Could you check a few things on this model? Use its own coordinates, in mm. A direction names the side the tool comes from. Round coordinates to 2 decimals unless told otherwise and drop trailing zeros. Write each loop counter-clockwise with the first axis right and the second up, starting at its lowest first coordinate (ties: lowest second). Pieces come first, ordered by that corner, then holes. Notation, with made-up numbers: (22, 34) -> (35, 34) arc R23 cw to (35, 70) -> close; hole circle Ø8 at (70.5, -1). An arc over 180 degrees is marked (long way). Return JSON: item names as keys, results as strings.
from build123d import *

# Parameters (mm, degrees)
F1_DEPTH  = 150
F2_R      = 13.1152364831
F3_DEPTH  = 30
F3_FACE_R = 13.1152364831
F4_DEPTH  = 15
F4_TAPER  = -65


with BuildPart() as f1:
    # F0 (on Front) → F1 (new body)
    with BuildSketch(Plane.XZ):
        Polygon((-24.6986329274, 10.7461681883), (3.0428618193, -26.762727648), (21.6557711081, 16.0165594597), align=None)
    extrude(amount=F1_DEPTH)

    # F2 (on Front) → F3 (join)
    with BuildSketch(Plane.XZ):
        Circle(F2_R)
    extrude(amount=-F3_DEPTH)

    # F3_face (on face) → F4 (join)
    with BuildSketch(Plane(origin=(0, 30, 0), x_dir=(1, 0, 0), z_dir=(0, 1, 0))):
        Circle(F3_FACE_R)
    extrude(amount=F4_DEPTH, taper=F4_TAPER)


solid = f1.part
1) For faces 4 (the face through (-2, -150, 0)), 5 (the face through (-10, 0, 9)), 6 (the face through (-11.02, -73.95, -7.75)), 7 (the face through (-1.197, -73.95, 13.418)), which set-ups out of +Z, -Z, +X, -X, +Y, -Y let a thin tool reach every point of the face, with its end or its side?
Return value:
{"face 4": "+Z, -Z, +X, -X, -Y", "face 5": "none", "face 6": "-Z, -X, -Y", "face 7": "+Z, -X, -Y"}
2) I want a section at B-B, the plane y = -111. Please give me the cut outline in (x, z).
Return value:
{"outline": "(-24.7, 10.75) -> (3.04, -26.76) -> (21.66, 16.02) -> close"}
3) I want a section at A-A, the plane x = 0. Please give me the cut outline in (y, z), and give its area (3 significant figures).
Return value:
{"outline": "(-150, -22.65) -> (0, -22.65) -> (0, -13.12) -> (30, -13.12) -> (45, -45.28) -> (45, 45.28) -> (30, 13.12) -> (0, 13.12) -> (0, 13.55) -> (-150, 13.55) -> close", "area": "7,090 mm²"}
4) Will these pins go through, and if not, where does the flat tip stop? pin 1 Ø3 at (y, z) = (-17.5, 4) entering from +X; pin 2 Ø10 at (y, z) = (-29.5, -23) entering from +X; pin 3 Ø3 at (x, y) = (18, -108) entering from +Z.
Return value:
{"pin 1": "x = 17.08", "pin 2": "x = 6.86", "pin 3": "z = 15.77"}
5) Thinking about a two-plate mould opening in Y: for faces 1 (the face through (-1, 45, -1)), 2 (the face through (12.22, -73.95, -5.67)), 3 (the face through (-1.707, 14.79, 13.004)), which applies, pulls with the +Y half, pulls with the -Y half, needs draft (parallel to the pull), parting line crosses it, or undercut?
Return value:
{"face 1": "pulls with the +Y half", "face 2": "needs draft", "face 3": "undercut"}
6) If I drill on probe 1 along Y at (x, z) = (-19, -33); probe 2 along X at (y, z) = (25.5, 1); probe 3 along Z at (x, y) = (-2, -17.5), over which ranges is the centre line in solid material (lowest first)? Write a range as [from, to].
Return value:
{"probe 1": "[41.64, 45]", "probe 2": "[-13.08, 13.08]", "probe 3": "[-19.94, 13.33]"}
